Check sheet for the drawn part. Datum: minimum x, y, z corner. Units: mm. Coordinates: 2 decimals unless noted, no trailing zeros. Loops run counter-clockwise (first coordinate to the right, second up) from the corner with the lowest first, then second, coordinate; pieces in that order, holes last. Notation, with made-up numbers: M -27,-13 L 7,-13 A23 ccw 7,14 Z; hole C 55.25,17 d1. An arc over 180 degrees is marked long. Use CSV: the item, a comma, the result in double quotes. Start each with the question number.
(1) Go/stop test with flat-tipped pins: pin 1 Ø21 at (x, y) = (310.5, 20.5) entering from +Z; pin 2 Ø11 at (x, z) = (206, 12.5) entering from +Y (3 decimals); pin 3 Ø12 at (x, z) = (248.5, 26) entering from -Y (3 decimals); pin 4 Ø5.5 at (x, y) = (6, 17.5) entering from +Z (3 decimals). Record where each tip stops, or that it passes through.
(2) Scan lines: line 1 (Y direction, x = 79, z = 6) (3 decimals); line 2 (X direction, y = 34.5, z = 9) (3 decimals); line 3 (X direction, y = 7.5, z = 4) (3 decimals). Record each from-to range of solid material in increasing order.
(3) Section check A-A on y = 34. Record the cut outline in (x, z) (3 decimals).
(4) Draft check along X on the marked faces 1 and 2. Enter one of: pulls with the +X half, pulls with the -X half, needs draft (parallel to the pull), parting line crosses it, or undercut.
(5) Section check D-D on z = 19.5. Record the cut outline in (x, y) (3 decimals).
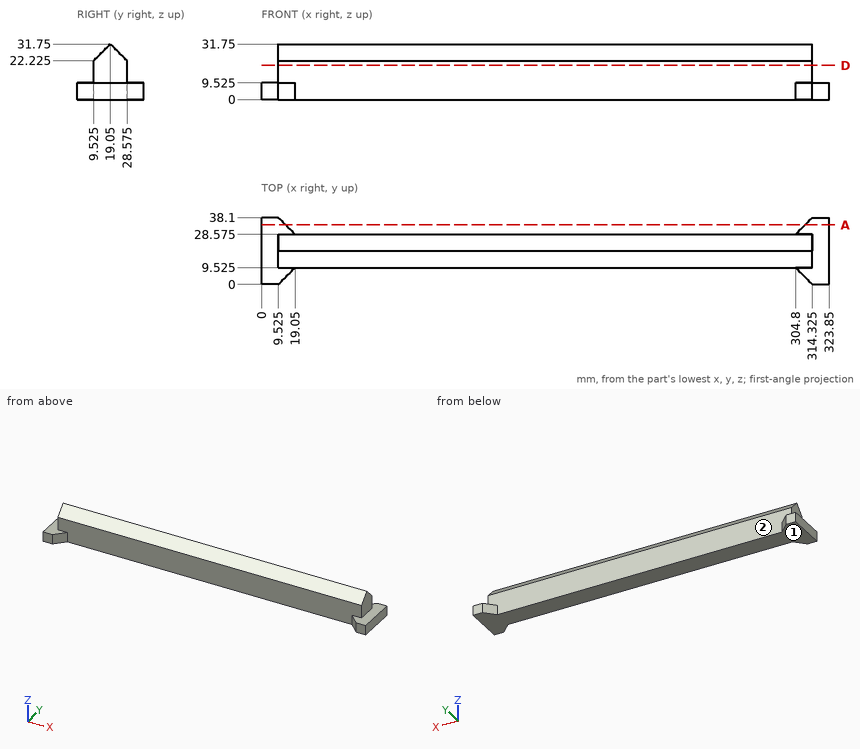
Outcome:
1,pin 1,"stops at z = 31.75"
1,pin 2,"stops at y = 28.575"
1,pin 3,"stops at y = 9.525"
1,pin 4,"stops at z = 9.525"
2,line 1,"y = 9.525 to 28.575"
2,line 2,"x = 0 to 13.125, 310.725 to 323.85"
2,line 3,"x = 0 to 17.025, 306.825 to 323.85"
3,outline,"M 0,0 L 13.625,0 L 13.625,9.525 L 0,9.525 Z; M 310.225,0 L 323.85,0 L 323.85,9.525 L 310.225,9.525 Z"
4,face 1,"needs draft"
4,face 2,"undercut"
5,outline,"M 9.525,9.525 L 314.325,9.525 L 314.325,28.575 L 9.525,28.575 Z"
